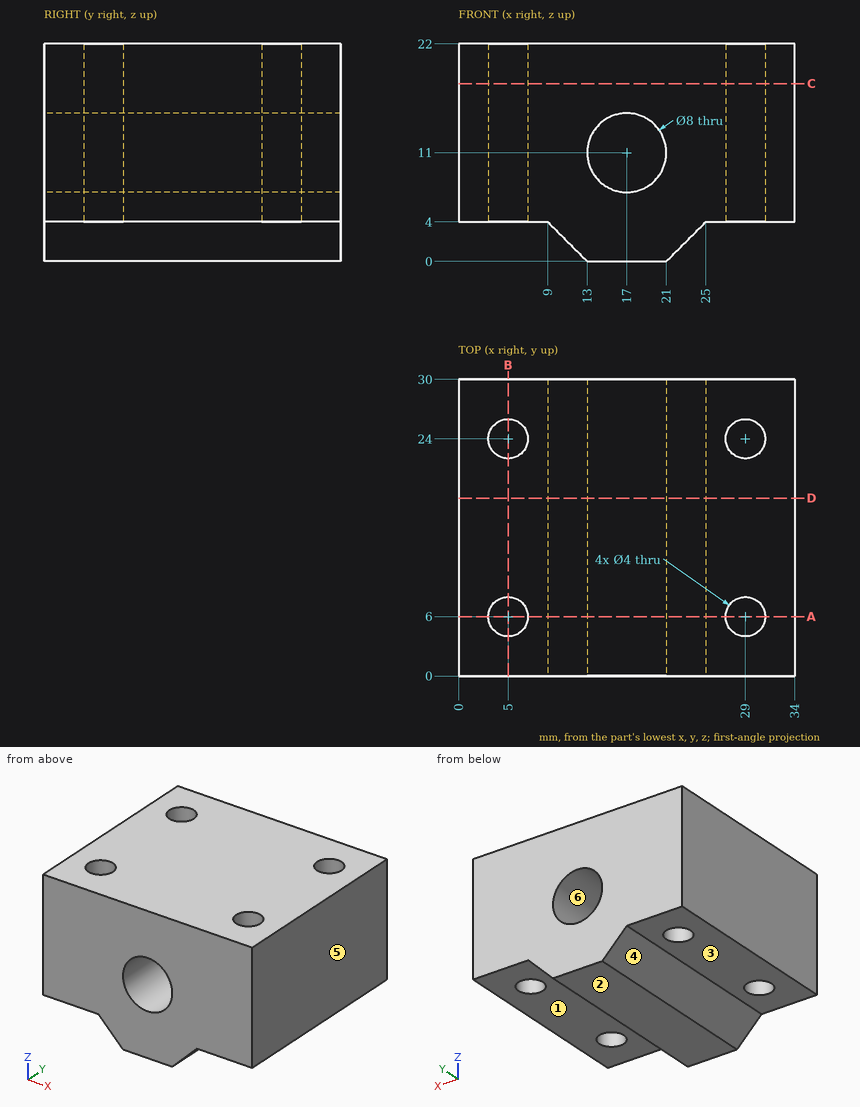
Check sheet for the drawn part. Datum: minimum x, y, z corner. Units: mm. A direction names the side the tool comes from. Round coordinates to 2 decimals unless told otherwise and drop trailing zeros. Write each loop counter-clockwise with the first axis right and the second up, starting at its lowest first coordinate (ties: lowest second). Pieces come first, ordered by that corner, then holes. Notation, with made-up numbers: (11, 82) -> (57, 82) arc R7 cw to (57, 88) -> close; hole circle Ø3 at (81.25, 83). An arc over 180 degrees is marked (long way). One line per item, written item: value. Start each with the question number.
(1) Cross-section at D-D, the plane y = 18. Record the cut outline in (x, z), and give its area (3 significant figures).
(2) Scan lines: line 1 (Y direction, x = 29, z = 18); line 2 (X direction, y = 24.25, z = 20.25); line 3 (Z direction, x = 28, y = 8.5). Record each from-to range of solid material in increasing order. Write a range as [from, to].
(3) Go/stop test with flat-tipped pins: pin 1 Ø3.5 at (x, y) = (5, 24) entering from -Z; pin 2 Ø4 at (y, z) = (14, 9) entering from -X; pin 3 Ø6.5 at (x, y) = (29, 24) entering from -Z; pin 4 Ø7 at (x, y) = (27.5, 18) entering from -Z. Record where each tip stops, or that it passes through.
(4) Cross-section at A-A, the plane y = 6. Record the cut outline in (x, z).
(5) Access from +Z, -Z, +X, -X, +Y, -Y to the whole of each face (thin tool, end or side, straight path). Record for the marked faces 1, 2 and 3.
(6) Draft check along Z on the marked faces 4, 5 and 6. Enter one of: +Z half, -Z half, draft (parallel to the pull), parting line (faces both ways), or undercut.
(7) Cross-section at C-C, the plane z = 18. Record the cut outline in (x, y).
(8) Cross-section at B-B, the plane x = 5. Record the cut outline in (y, z), and give its area (3 significant figures).
Answer:
1. outline: (0, 4) -> (9, 4) -> (13, 0) -> (21, 0) -> (25, 4) -> (34, 4) -> (34, 22) -> (0, 22) -> close; hole circle Ø8 at (17, 11)
1. area: 610 mm²
2. line 1: [0, 4], [8, 22], [26, 30]
2. line 2: [0, 3.02], [6.98, 27.02], [30.98, 34]
2. line 3: [4, 22]
3. pin 1: through
3. pin 2: x = 0
3. pin 3: z = 4
3. pin 4: z = 3
4. outline: (0, 4) -> (3, 4) -> (3, 22) -> (0, 22) -> close; (7, 4) -> (9, 4) -> (13, 0) -> (21, 0) -> (25, 4) -> (27, 4) -> (27, 22) -> (7, 22) -> close; (31, 4) -> (34, 4) -> (34, 22) -> (31, 22) -> close; hole circle Ø8 at (17, 11)
5. face 1: -Z, +X, +Y, -Y
5. face 2: -Z, +X, -X, +Y, -Y
5. face 3: -Z, -X, +Y, -Y
6. face 4: -Z half
6. face 5: draft
6. face 6: undercut
7. outline: (0, 0) -> (34, 0) -> (34, 30) -> (0, 30) -> close; hole circle Ø4 at (5, 6); hole circle Ø4 at (5, 24); hole circle Ø4 at (29, 6); hole circle Ø4 at (29, 24)
8. outline: (0, 4) -> (4, 4) -> (4, 22) -> (0, 22) -> close; (8, 4) -> (22, 4) -> (22, 22) -> (8, 22) -> close; (26, 4) -> (30, 4) -> (30, 22) -> (26, 22) -> close
8. area: 396 mm²
